Could you check a few things on this drawing? It's one solid part, dimensions in mm from its lowest x, y, z. Round coordinates to 2 decimals unless told otherwise and drop trailing zeros. Loops run counter-clockwise (first coordinate to the right, second up) from the corner with the lowest first, then second, coordinate; pieces in that order, holes last. Notation, with made-up numbers: M 13,72.25 L 61,72.25 A15 ccw 61,98.25 Z; hole C -20,-13 d1. An arc over 180 degrees is marked long. Write item = value, one per line. Start each with the question number.
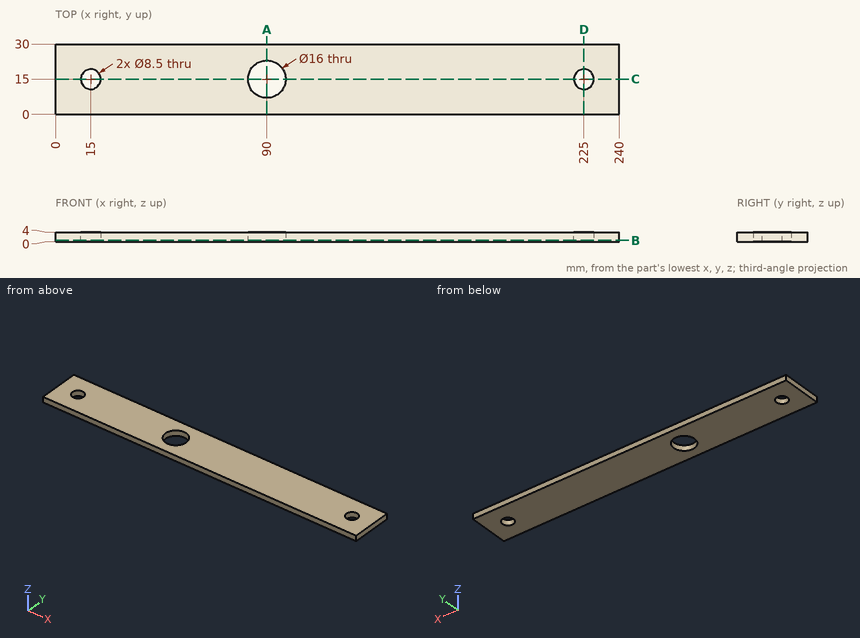
Item 1: I want a section at C-C, the plane y = 15. List the corners of the cut face in (x, z) for me, then the cut area to 3 significant figures.
Item 2: I want a section at A-A, the plane x = 90. List the corners of the cut face in (y, z) for me, then the cut area to 3 significant figures.
Item 3: Please list where these lines run through material, in increasing order: line 1 (X direction, y = 15.5, z = 2.35); line 2 (Y direction, x = 15, z = 1.95); line 3 (Y direction, x = 90, z = 2.4). Write a range as [from, to].
Item 4: I want a section at B-B, the plane z = 0.6. List the corners of the cut face in (x, y) for me, then the cut area to 3 significant figures.
Item 5: I want a section at D-D, the plane x = 225. List the corners of the cut face in (y, z) for me.
Worked out:
q1.outline = M 0,0 L 10.75,0 L 10.75,4 L 0,4 Z; M 19.25,0 L 82,0 L 82,4 L 19.25,4 Z; M 98,0 L 220.75,0 L 220.75,4 L 98,4 Z; M 229.25,0 L 240,0 L 240,4 L 229.25,4 Z
q1.area = 828 mm2
q2.outline = M 0,0 L 7,0 L 7,4 L 0,4 Z; M 23,0 L 30,0 L 30,4 L 23,4 Z
q2.area = 56.0 mm2
q3.line_1 = [0, 10.78], [19.22, 82.02], [97.98, 220.78], [229.22, 240]
q3.line_2 = [0, 10.75], [19.25, 30]
q3.line_3 = [0, 7], [23, 30]
q4.outline = M 0,0 L 240,0 L 240,30 L 0,30 Z; hole C 15,15 d8.5; hole C 90,15 d16; hole C 225,15 d8.5
q4.area = 6,890 mm2
q5.outline = M 0,0 L 10.75,0 L 10.75,4 L 0,4 Z; M 19.25,0 L 30,0 L 30,4 L 19.25,4 Z
